Read the model definition and answer for the solid it produces. Units are mm, in the model's axes. Face numbers are marked on the shaded views. A direction names the side the tool comes from. Coordinates: 2 decimals unless noted, no trailing zeros. Write each loop counter-clockwise with the first axis right and the second up, starting at its lowest first coordinate (ties: lowest second). Pieces come first, ordered by that corner, then holes. Notation, with made-up numbers: (32, -29) -> (42, -29) arc R4 cw to (42, -24) -> close; hole circle Ø3 at (29.5, 35). An arc over 180 degrees is marked (long way). Answer as a JSON object with one key per item and string values. Group by question number.
(1) Find section B-B (x = 292.5). Give the vertices of the cut face in (y, z), then the cut area to 3 significant figures.
(2) Find section D-D (z = 45). Give the vertices of the cut face in (x, y).
(3) Find section C-C (x = 63.5). Give the vertices of the cut face in (y, z), then the cut area to 3 significant figures.
(4) Flat-ended cylindrical pins translate along their axes: P1, Ø20, axis at x = 9, z = 174.5, coming from the -Y side; P2, Ø5, axis at y = -36.5, z = -22.5, coming from the +X side; P3, Ø4, axis at y = 9, z = 164, coming from the +X side. Find the tip coordinate at first contact, or state that the pin passes through.
(5) Which of the six approach directions +Z, -Z, +X, -X, +Y, -Y give full straight-line access (tool end or side, diameter ignored) to the marked faces 3 and 4?
(6) Straight lines are drawn through the part: L1, parallel to Y at x = 292, z = -27; L2, parallel to X at y = -87, z = -26; L3, parallel to Z at x = 53, y = 1. For each, find the intervals that lie inside material, in ascending order.
(7) For a pull along Z with two mould halves and no side action, classify the marked faces 1 and 2 as +Z half, -Z half, draft (parallel to the pull), parting line (faces both ways), or undercut.
(8) Find section A-A (y = -87.5). Give the vertices of the cut face in (x, z), then the cut area to 3 significant figures.
Autodesk Inventor part; units mm, degrees
ref_plane "YZ Plane" through (0, 0, 0) normal (1, 0, 0) x (0, 1, 0)
ref_plane "XZ Plane" through (0, 0, 0) normal (0, 1, 0) x (-1, 0, 0)
ref_plane "XY Plane" through (0, 0, 0) normal (0, 0, 1) x (1, 0, 0)
sketch "Skizze1" plane through (0, 0, 0) normal (0, 0, 1) x (1, 0, 0)
  circle A0 centre (0, 0) radius 12.45
  dimension "d0" = 24.9
extrude "Extrusion1" add sketch "Skizze1" along normal blind 50
sketch "Skizze2" plane through (0, 0, 50) normal (0, 0, 1) x (1, 0, 0)
  circle A0 centre (0, 0) radius 17.5
  dimension "d3" = 35
extrude "Extrusion2" add sketch "Skizze2" along normal blind 10
sketch "Skizze3" plane through (0, 0, 0) normal (0, 0, -1) x (-1, 0, 0)
  circle A0 centre (0, 0) radius 17.5
  dimension "d6" = 35
extrude "Extrusion3" add sketch "Skizze3" along normal blind 10
sketch "Skizze4" plane through (0, 0, -10) normal (0, 0, -1) x (-1, 0, 0)
  circle A0 centre (0, 0) radius 12.5
  dimension "d9" = 25
extrude "Extrusion4" add sketch "Skizze4" along normal blind 10
sketch "Skizze5" plane through (0, 0, 60) normal (0, 0, 1) x (1, 0, 0)
  circle A0 centre (0, 0) radius 12.5
  dimension "d12" = 25
extrude "Extrusion5" add sketch "Skizze5" along normal blind 100
sketch "Skizze6" plane through (0, 0, -20) normal (0, 0, -1) x (-1, 0, 0)
  line L0 (-12.5, 0) -> (12.5, 0)
  line L1 (12.5, 0) -> (12.5, -100)
  line L2 (12.5, -100) -> (-12.5, -100)
  line L3 (-12.5, -100) -> (-12.5, 0)
  circle A0 centre (0, 0) radius 17.5
  arc A1 (12.5, 0) -> (-12.5, 0) centre (0, 0) ccw
  line L4 (0, 0) -> (12.5, 0) construction
  line L5 (0, 0) -> (-12.5, 0) construction
  dimension "d15" = 25
  dimension "d16" = 12.5
  dimension "d17" = 0
  dimension "d18" = 100
  dimension "d19" = 180
extrude "Extrusion6" add sketch "Skizze6" along normal blind 10 contours A1 L0 | L0 L1 A0 L3 | A0 L1 L2 L3
sketch "Skizze8" plane through (0, 0, -30) normal (0, 0, -1) x (-1, 0, 0)
  line L0 (-12.5, -100) -> (-302.5, -100)
  line L1 (-302.5, -100) -> (-302.5, -75)
  line L2 (-302.5, -75) -> (-12.5, -75)
  line L3 (-12.5, -75) -> (-12.5, -100)
  line L4 (-12.5, 0) -> (-12.5, -100)
  line L5 (-12.5, -100) -> (12.5, -100)
  point P0 (0, 0)
  dimension "d23" = 25
  dimension "d24" = 0
  dimension "d26" = 290
  dimension "d29" = 0
extrude "Extrusion7" add sketch "Skizze8" against normal blind 10
sketch "Skizze9" plane through (0, 0, -20) normal (0, 0, 1) x (1, 0, 0)
  circle A0 centre (292.5, -87.5) radius 6
  line L0 (302.5, -100) -> (302.5, -75)
  line L1 (-12.5, -100) -> (302.5, -100)
  point P0 (0, 0)
  dimension "d30" = 12
  dimension "d31" = 10
  dimension "d32" = 12.5
extrude "Extrusion8" cut sketch "Skizze9" against normal up to surface (10 mm away)
sketch "Skizze10" plane through (0, 0, 160) normal (0, 0, 1) x (1, 0, 0)
  line L0 (150, -12.5) -> (-150, -12.5)
  line L1 (-150, -12.5) -> (-150, 12.5)
  line L2 (-150, 12.5) -> (150, 12.5)
  line L3 (150, 12.5) -> (150, -12.5)
  point P0 (0, 0)
  dimension "d35" = 25
  dimension "d36" = 12.5
  dimension "d37" = 300
  dimension "d38" = 150
extrude "Extrusion9" add sketch "Skizze10" along normal blind 25
sketch "Skizze11" plane through (150, -12.5, 160) normal (1, 0, 0) x (0, 0, -1)
  line L0 (0, 0) -> (-25, 0)
  line L1 (-25, 25) -> (-25, 0)
  line L2 (0, 0) -> (-25, 0)
  line L3 (-25, 0) -> (-25, 25)
  line L4 (-25, 25) -> (0, 25)
  line L5 (0, 25) -> (0, 0)
  circle A0 centre (-12.5, 12.5) radius 12.5
  point P0 (160, 12.5)
  point P1 (-25, 12.5)
  point P2 (-12.5, 25)
  point P3 (0, 12.5)
  point P4 (-12.5, 0)
extrude "Extrusion10" cut sketch "Skizze11" against normal blind 120 contours L0 A0 L5 | L0 L1 A0 | A0 L4 L5 | L1 L4 A0
sketch "Skizze12" plane through (-150, -12.5, 160) normal (-1, 0, 0) x (0, 0, 1)
  line L0 (0, 25) -> (25, 25)
  line L1 (0, 0) -> (25, 0)
  line L2 (25, 0) -> (25, 25)
  line L3 (25, 25) -> (0, 25)
  line L4 (0, 25) -> (0, 0)
  circle A0 centre (12.5, 12.5) radius 12.5
  point P0 (-160, 12.5)
  point P1 (12.5, 25)
  point P2 (25, 12.5)
  point P3 (12.5, 0)
  point P4 (0, 12.5)
extrude "Extrusion11" cut sketch "Skizze12" against normal blind 120 contours L0 A0 L4 | L0 L2 A0 | A0 L1 L4 | L2 L1 A0
properties part number "Lenkung_vorne"
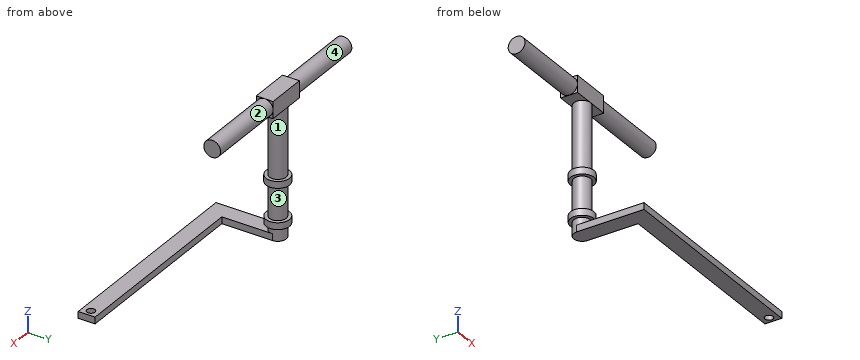
Results below:
{
 "1": {"outline": "(-100, -30) -> (-93.5, -30) -> (-93.5, -20) -> (-100, -20) -> close; (-81.5, -30) -> (-75, -30) -> (-75, -20) -> (-81.5, -20) -> close", "area": "130 mm2"},
 "2": {"outline": "circle Ø24.9 at (0, 0)"},
 "3": {"outline": "(-100, -30) -> (-75, -30) -> (-75, -20) -> (-100, -20) -> close; circle Ø25 at (0, 172.5)", "area": "741 mm2"},
 "4": {"P1": "stops at y = -12.5", "P2": "stops at x = 12.5", "P3": "stops at x = 150"},
 "5": {"face 3": "none", "face 4": "-X"},
 "6": {"L1": "y = -100 to -93.48, -81.52 to -75", "L2": "x = -12.5 to 286.52, 298.48 to 302.5", "L3": "z = 160.04 to 184.96"},
 "7": {"face 1": "undercut", "face 2": "parting line"},
 "8": {"outline": "(-12.5, -30) -> (286.5, -30) -> (286.5, -20) -> (-12.5, -20) -> close; (298.5, -30) -> (302.5, -30) -> (302.5, -20) -> (298.5, -20) -> close", "area": "3,030 mm2"}
}
